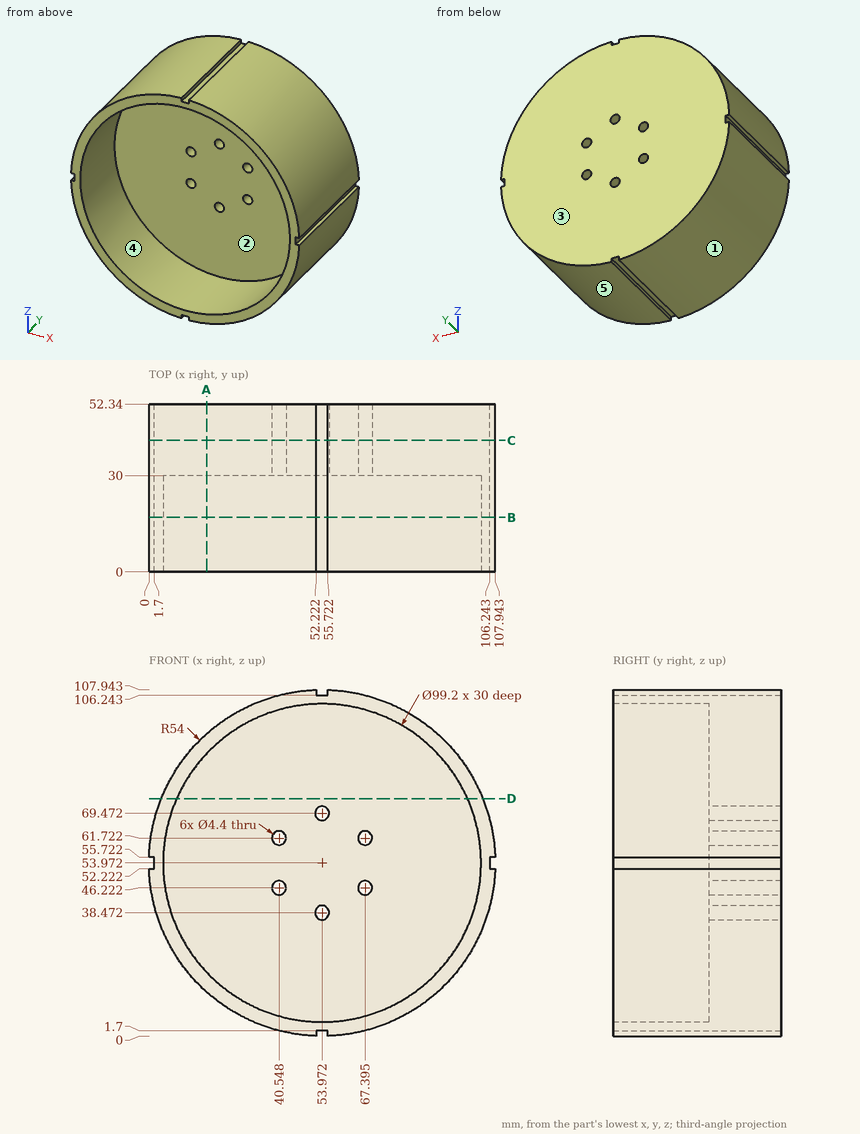
For this review, use the dimensioned drawing (mm, ordinates from the lowest corner) and the shaded views. A direction names the side the tool comes from. Give positions to 0.01 mm unless a question says otherwise; leave off trailing zeros. Write each loop counter-clockwise with the first axis right and the second up, starting at its lowest first coordinate (ties: lowest second). Pieces come first, ordered by that corner, then holes. Notation, with made-up numbers: M 62.25,68.25 L 121.25,68.25 A15 cw 121.25,92.25 Z; hole C -12,85 d8. An arc over 180 degrees is marked long. Answer as a JSON object with one key per item and string values. Group by question number.
Item 1: Tool access review of the marked faces 1 and 2: name each direction out of +Z, -Z, +X, -X, +Y, -Y from which nothing blocks a thin tool from reaching the whole face with its end or side.
Item 2: For pin 1 Ø1.5 at (x, y) = (93.5, 12) entering from +Z; pin 2 Ø10 at (x, y) = (63, 36.5) entering from +Z; pin 3 Ø10 at (x, y) = (12.5, 11) entering from +Z (1 decimal), all flat-tipped, find the tip position at first contact; note any pin that passes through.
Item 3: Consider section C-C on y = 41. Write out the cut boundary in (x, z) (1 decimal), plus the area to 3 significant figures.
Item 4: Draft analysis for pull direction X (two halves, no side actions). For the marked faces 3, 4 and 5, state which applies: +X half, -X half, draft (parallel to the pull), parting line (faces both ways), or undercut.
Item 5: Consider section B-B on y = 17. Write out the cut boundary in (x, z).
Item 6: Consider section A-A on x = 18. Write out the cut boundary in (y, z), plus the area to 3 significant figures.
Item 7: Consider section D-D on z = 74. Write out the cut boundary in (x, y) (1 decimal).
Item 8: For probe 1 along X at (y, z) = (32.5, 44.5) (1 decimal); probe 2 along Y at (x, z) = (58.5, 100); probe 3 along Z at (x, y) = (78.5, 10) (1 decimal), list the stretches that pass through material, from the lowest coordinate up. Write a range as [from, to].
Check result:
{
 "1": {"face 1": "-Z, -X, +Y, -Y", "face 2": "-Y"},
 "2": {"pin 1": "stops at z = 91.55", "pin 2": "stops at z = 107.82", "pin 3": "stops at z = 93.8"},
 "3": {"outline": "M 0,52.2 A54 ccw 52.2,0 L 52.2,1.7 L 55.7,1.7 L 55.7,0 A54 ccw 107.9,52.2 L 106.2,52.2 L 106.2,55.7 L 107.9,55.7 A54 ccw 55.7,107.9 L 55.7,106.2 L 52.2,106.2 L 52.2,107.9 A54 ccw 0,55.7 L 1.7,55.7 L 1.7,52.2 Z; hole C 40.5,46.2 d4.4; hole C 40.5,61.7 d4.4; hole C 54,38.5 d4.4; hole C 54,69.5 d4.4; hole C 67.4,46.2 d4.4; hole C 67.4,61.7 d4.4", "area": "9,050 mm^2"},
 "4": {"face 3": "draft", "face 4": "undercut", "face 5": "+X half"},
 "5": {"outline": "M 0,52.22 A54 ccw 52.22,0 L 52.22,1.7 L 55.72,1.7 L 55.72,0 A54 ccw 107.94,52.22 L 106.24,52.22 L 106.24,55.72 L 107.94,55.72 A54 ccw 55.72,107.94 L 55.72,106.24 L 52.22,106.24 L 52.22,107.94 A54 ccw 0,55.72 L 1.7,55.72 L 1.7,52.22 Z; hole C 53.97,53.97 d99.2"},
 "6": {"outline": "M 0,13.7 L 52.34,13.7 L 52.34,94.25 L 0,94.25 L 0,88.12 L 30,88.12 L 30,19.82 L 0,19.82 Z", "area": "2,170 mm^2"},
 "7": {"outline": "M 3.8,0 L 8.6,0 L 8.6,30 L 99.3,30 L 99.3,0 L 104.1,0 L 104.1,52.3 L 3.8,52.3 Z"},
 "8": {"probe 1": "x = [0.8, 39.2], [41.9, 66], [68.8, 107.1]", "probe 2": "y = [30, 52.34]", "probe 3": "z = [5.9, 10.9], [97.1, 102.1]"}
}
